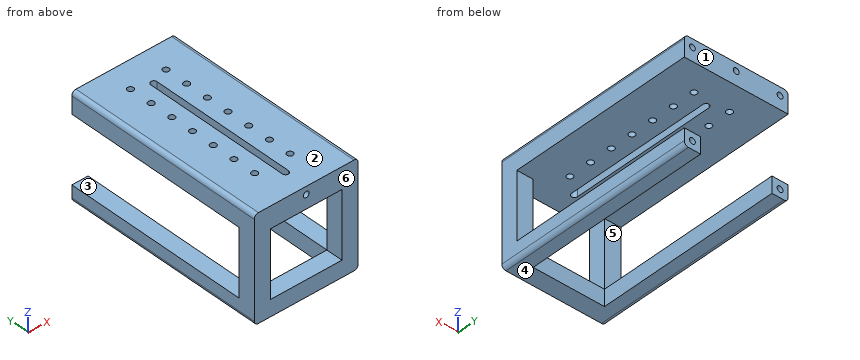
Autodesk Inventor part; units mm, degrees
ref_plane "YZ Plane" through (0, 0, 0) normal (1, 0, 0) x (0, 1, 0)
ref_plane "XZ Plane" through (0, 0, 0) normal (0, 1, 0) x (-1, 0, 0)
ref_plane "XY Plane" through (0, 0, 0) normal (0, 0, 1) x (1, 0, 0)
sketch "Sketch1" plane through (0, 0, 0) normal (0, 1, 0) x (-1, 0, 0)
  line L0 (0, 0) -> (49.8, 0)
  line L1 (49.8, 0) -> (49.8, -49.8)
  line L2 (49.8, -49.8) -> (0, -49.8)
  line L3 (0, -49.8) -> (0, 0)
  line L4 (7.8, -7.8) -> (42, -7.8)
  line L5 (42, -7.8) -> (42, -42)
  line L6 (42, -42) -> (7.8, -42)
  line L7 (7.8, -42) -> (7.8, -7.8)
  dimension "d0" = 49.8
  dimension "d1" = 49.8
  dimension "d2" = 7.8
extrude "Extrusion1" add sketch "Sketch1" along normal blind 8
sketch "Sketch3" plane through (0, 0, 0) normal (0, -1, 0) x (1, 0, 0)
  line L0 (-49.8, 0) -> (0, 0)
  line L1 (-49.8, -49.8) -> (-49.8, 0)
  line L2 (0, 0) -> (-49.8, 0)
  line L3 (-49.8, 0) -> (-49.8, -10.23)
  line L4 (-49.8, -10.23) -> (0, -10.23)
  line L5 (0, -10.23) -> (0, 0)
  line L6 (-7.8, -42) -> (-7.8, -7.8)
  line L7 (0, -49.8) -> (-7.8, -49.8)
  line L8 (-7.8, -49.8) -> (-7.8, -42)
  line L9 (-7.8, -42) -> (0, -42)
  line L10 (0, -42) -> (0, -49.8)
  line L11 (0, -49.8) -> (-49.8, -49.8)
  line L12 (-42, -7.8) -> (-42, -42)
  line L13 (-49.8, -49.8) -> (-42, -49.8)
  line L14 (-42, -49.8) -> (-42, -42)
  line L15 (-42, -42) -> (-49.8, -42)
  line L16 (-49.8, -42) -> (-49.8, -49.8)
  dimension "d6" = 10.23
extrude "Extrusion2" add sketch "Sketch3" against normal blind 97 contours L0 L5 L4 L1 | L15 L14 L11 L1 | L9 L10 L7 L8
sketch "Sketch4" plane through (-49.8, 0, 0) normal (0, 0, 1) x (1, 0, 0)
  line L0 (23.45, 81) -> (26.35, 81)
  line L1 (26.35, 81) -> (26.35, 11)
  line L2 (26.35, 11) -> (23.45, 11)
  line L3 (23.45, 11) -> (23.45, 81)
  line L4 (49.8, 0) -> (49.8, 97)
  line L5 (0, 0) -> (49.8, 0)
  circle A0 centre (24.9, 81) radius 1.45
  circle A1 centre (24.9, 11) radius 1.45
  circle A2 centre (16.4, 84) radius 1.45
  circle A3 centre (33.4, 84) radius 1.45
  line L6 (0, 97) -> (49.8, 97)
  circle A4 centre (16.4, 73) radius 1.45
  circle A5 centre (33.4, 73) radius 1.45
  circle A6 centre (16.4, 62) radius 1.45
  circle A7 centre (33.4, 62) radius 1.45
  circle A8 centre (16.4, 51) radius 1.45
  circle A9 centre (33.4, 51) radius 1.45
  circle A10 centre (16.4, 40) radius 1.45
  circle A11 centre (33.4, 40) radius 1.45
  circle A12 centre (16.4, 29) radius 1.45
  circle A13 centre (33.4, 29) radius 1.45
  circle A14 centre (16.4, 18) radius 1.45
  circle A15 centre (33.4, 18) radius 1.45
  dimension "d9" = 2.9
  dimension "d10" = 70
  dimension "d11" = 23.45
  dimension "d12" = 11
  dimension "d15" = 2.9
  dimension "d16" = 7.05
  dimension "d17" = 2.9
  dimension "d18" = 7.05
  dimension "d19" = 13
  dimension "d20" = 13
  dimension "d23" = 11
extrude "Extrusion3" cut sketch "Sketch4" against normal through all
sketch "Sketch5" plane through (0, 97, 0) normal (0, 1, 0) x (1, 0, 0)
  circle A0 centre (-45.9, 45.9) radius 1.4
  circle A1 centre (-3.9, 45.9) radius 1.4
  line L0 (-49.8, 49.8) -> (-49.8, 0)
  line L1 (-49.8, 24.9) -> (-42, 24.9)
  line L2 (-42, 10.23) -> (-42, 42)
  circle A2 centre (-45.9, 3.9) radius 1.4
  circle A3 centre (-3.9, 3.9) radius 1.4
  point P0 (0, 0)
  dimension "d28" = 2.8
  dimension "d29" = 2.8
extrude "Extrusion4" cut sketch "Sketch5" against normal blind 20
sketch "Sketch6" plane through (0, 0, 0) normal (0, -1, 0) x (1, 0, 0)
  line L0 (-49.8, 0) -> (0, 0)
  circle A0 centre (-24.9, -3.7) radius 1.4
  line L1 (-49.8, -49.8) -> (-49.8, 0)
  dimension "d37" = 2.8
  dimension "d38" = 3.7
  dimension "d39" = 24.9
extrude "Extrusion5" cut sketch "Sketch6" against normal blind 10
fillet "Fillet1" radius 2 4 edges at (0, 48.5, 0) (0, 48.5, -49.8) (-49.8, 48.5, -49.8) (-49.8, 48.5, 0)
sketch "Sketch7" plane through (0, 97, 0) normal (0, 1, 0) x (1, 0, 0)
  circle A0 centre (-24.9, 3.7) radius 1.4
  circle A1 centre (-24.9, 3.7) radius 1.4
  point P0 (0, 0)
extrude "Extrusion6" cut sketch "Sketch7" against normal blind 10
properties part number "00_Linear_Stage_NEMA11_Mount"
Build history of the part. All positions in model axes, mm. Face numbers are marked on the shaded views. A direction names the side the tool comes from. Give positions to 0.01 mm unless a question says otherwise; leave off trailing zeros. Order: outer loops, then holes, each group sorted by start corner. A loop starts at its lowest first (then second) coordinate and runs counter-clockwise, first axis right, second up. Notation, with made-up numbers: M 63.5,85 L 103.5,85 A31 cw 103.5,124 Z; hole C -27,5.25 d9. An arc over 180 degrees is marked long. Use one line per item in the form item = value.
Q1. Pin check, flat tips, straight feed: P1, Ø12, axis at y = 48, z = -17.5, coming from the +X side; P2, Ø8.5, axis at x = -48, z = -31.5, coming from the +Y side; P3, Ø12, axis at x = -26, y = 35, coming from the -Z side; P4, Ø2, axis at x = -24.9, z = -3.7, coming from the +Y side. Stop position of each tip, or through.
Conclusion:
P1 = through
P2 = 8
P3 = -10.23
P4 = 87
Q2. Slice it at A-A, the plane y = 84. State how many separate pieces and enclosed holes the cut face has, and give its area (3 significant figures).
Conclusion:
separate_pieces = 5
enclosed_holes = 4
area = 544 mm2
Q3. Slice it at B-B, the plane x = -12. Write the cut outline in (y, z), and give its area (3 significant figures).
Conclusion:
outline = M 0,-49.8 L 8,-49.8 L 8,-42 L 0,-42 Z; M 0,-10.23 L 97,-10.23 L 97,0 L 0,0 Z
area = 1,050 mm2
Q4. Slice it at D-D, the plane y = 40. Write the cut outline in (x, z).
Conclusion:
outline = M -49.8,-47.8 A2 ccw -47.8,-49.8 L -42,-49.8 L -42,-42 L -49.8,-42 Z; M -49.8,-10.23 L -34.85,-10.23 L -34.85,0 L -47.8,0 A2 ccw -49.8,-2 Z; M -31.95,-10.23 L -26.35,-10.23 L -26.35,0 L -31.95,0 Z; M -23.45,-10.23 L -17.85,-10.23 L -17.85,0 L -23.45,0 Z; M -14.95,-10.23 L 0,-10.23 L 0,-2 A2 ccw -2,0 L -14.95,0 Z; M -7.8,-49.8 L -2,-49.8 A2 ccw 0,-47.8 L 0,-42 L -7.8,-42 Z
Q5. Which spindle directions (+Z, -Z, +X, -X, +Y, -Y) get a long thin tool onto all of the face, cutting with end or side? Do the marked faces 5 and 6. Say none if no direction does.
Conclusion:
face_5 = +X, -X, +Y
face_6 = +Z, -Z, +X, -X, -Y
Q6. Pull direction Z, two halves, no side cores. Call the marked faces 1, 2, 3 and 4: released by +Z, released by -Z, zero draft, split by the parting line, or undercut.
Conclusion:
face_1 = zero draft
face_2 = released by +Z
face_3 = undercut
face_4 = released by -Z
Q7. Wall check: probe 1 along Z at (x, y) = (-45.9, 81); probe 2 along X at (y, z) = (90, -3); probe 3 along Z at (x, y) = (-7, 36). Give the ranges that are in metal, low to high.
Conclusion:
probe_1 = -49.8 to -47.3, -44.5 to -42, -10.23 to -5.3, -2.5 to 0
probe_2 = -49.8 to -46.97, -44.83 to -26.11, -23.69 to -4.97, -2.83 to 0
probe_3 = -49.8 to -42, -10.23 to 0
Q8. Slice it at C-C, the plane z = -41. Write the cut outline in (x, y).
Conclusion:
outline = M -49.8,0 L -42,0 L -42,8 L -49.8,8 Z; M -7.8,0 L 0,0 L 0,8 L -7.8,8 Z
